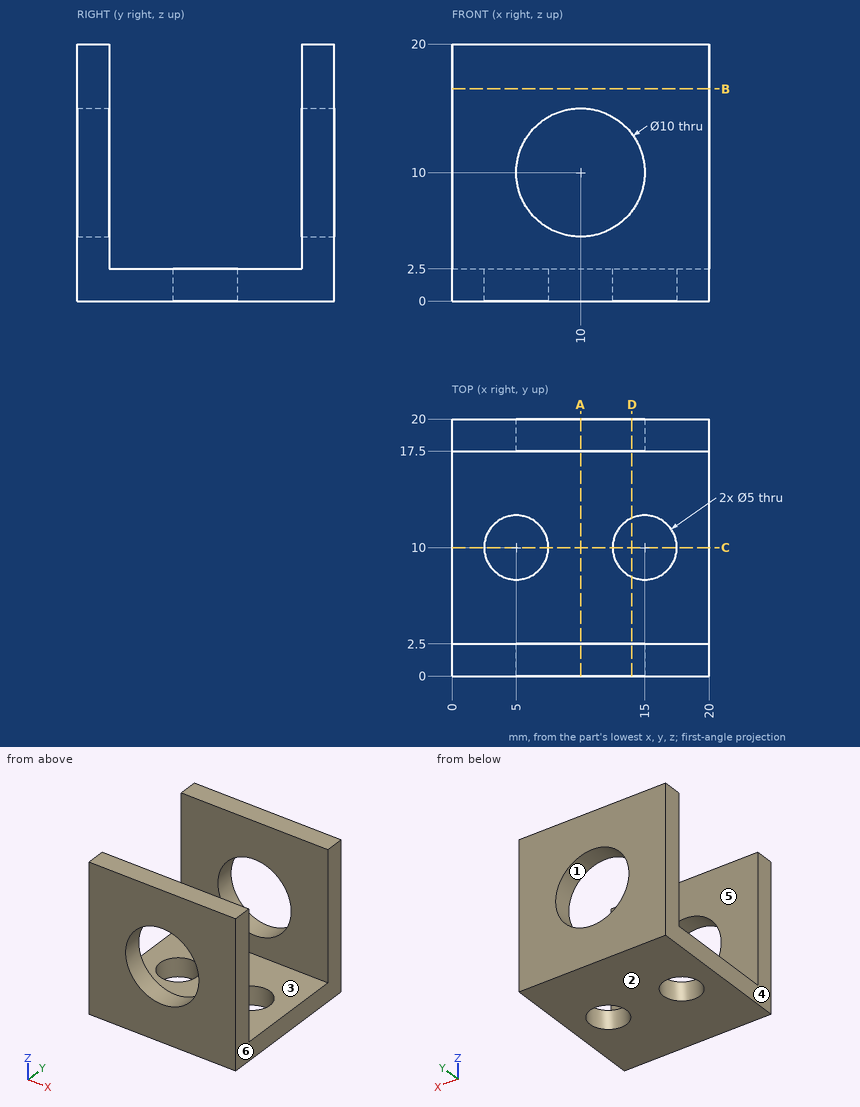
Could you check a few things on this drawing? It's one solid part, dimensions in mm from its lowest x, y, z. A direction names the side the tool comes from. Give positions to 0.01 mm unless a question says otherwise; leave off trailing zeros. Order: outer loops, then holes, each group sorted by start corner. A loop starts at its lowest first (then second) coordinate and runs counter-clockwise, first axis right, second up. Notation, with made-up numbers: (30, 60) - (82, 60) arc R25 ccw to (82, 72) - close; hole circle Ø3 at (-31, 74.5). An arc over 180 degrees is marked (long way). One line per question, with ' | ' between items. Start each with the question number.
Item 1: I want a section at D-D on x = 14. Write out the boundary of the cut face in (y, z), then the cut area to 3 significant figures.
Item 2: I need wall thicknesses on probe 1 along Y at (x, z) = (5, 1.6); probe 2 along Z at (x, y) = (10, 1.35); probe 3 along Y at (x, z) = (6.25, 17). Which ranges of each line are inside material? Lowest first, please. Write a range as [from, to].
Item 3: I want a section at A-A on x = 10. Write out the boundary of the cut face in (y, z), then the cut area to 3 significant figures.
Item 4: I want a section at B-B on z = 16.5. Write out the boundary of the cut face in (x, y), then the cut area to 3 significant figures.
Item 5: I'm going to push a flat-ended pin straight in: pin 1 Ø1.5 at (x, y) = (7.5, 4.5) entering from +Z. Where does the tip first touch, or does it pass through?
Item 6: I want a section at C-C on y = 10. Write out the boundary of the cut face in (x, z).
Item 7: For the marked faces 5 and 6, which set-ups out of +Z, -Z, +X, -X, +Y, -Y let a thin tool reach every point of the face, with its end or its side?
Item 8: Thinking about a two-plate mould opening in Z: for the marked faces 1, 2, 3 and 4, which applies, pulls with the +Z half, pulls with the -Z half, needs draft (parallel to the pull), parting line crosses it, or undercut?
Verdict:
1) outline: (0, 0) - (7.71, 0) - (7.71, 2.5) - (2.5, 2.5) - (2.5, 7) - (0, 7) - close; (0, 13) - (2.5, 13) - (2.5, 20) - (0, 20) - close; (12.29, 0) - (20, 0) - (20, 7) - (17.5, 7) - (17.5, 2.5) - (12.29, 2.5) - close; (17.5, 13) - (20, 13) - (20, 20) - (17.5, 20) - close | area: 96.0 mm^2
2) probe 1: [0, 7.5], [12.5, 20] | probe 2: [0, 5], [15, 20] | probe 3: [0, 2.5], [17.5, 20]
3) outline: (0, 0) - (20, 0) - (20, 5) - (17.5, 5) - (17.5, 2.5) - (2.5, 2.5) - (2.5, 5) - (0, 5) - close; (0, 15) - (2.5, 15) - (2.5, 20) - (0, 20) - close; (17.5, 15) - (20, 15) - (20, 20) - (17.5, 20) - close | area: 87.5 mm^2
4) outline: (0, 0) - (20, 0) - (20, 2.5) - (0, 2.5) - close; (0, 17.5) - (20, 17.5) - (20, 20) - (0, 20) - close | area: 100 mm^2
5) pin 1: z = 2.5
6) outline: (0, 0) - (2.5, 0) - (2.5, 2.5) - (0, 2.5) - close; (7.5, 0) - (12.5, 0) - (12.5, 2.5) - (7.5, 2.5) - close; (17.5, 0) - (20, 0) - (20, 2.5) - (17.5, 2.5) - close
7) face 5: +Z, +X, -X | face 6: +Z, -Z, +X, +Y, -Y
8) face 1: undercut | face 2: pulls with the -Z half | face 3: pulls with the +Z half | face 4: needs draft
